Verification items for the finished model (mm, model axes). A direction names the side the tool comes from. Give positions to 0.01 mm unless a question says otherwise; leave off trailing zeros. Loops run counter-clockwise (first coordinate to the right, second up) from the corner with the lowest first, then second, coordinate; pieces in that order, holes last. Notation, with made-up numbers: (31, 12) - (51, 12) arc R22 cw to (51, 18) - close; hole circle Ø3 at (32, 88.5). An arc over 180 degrees is marked (long way). One line per question, with ' | ' between items. Start each with the question number.
1. Section check C-C, the plane y = 7. Enter the section's corners in (x, z).
2. Section check A-A, the plane y = 29. Enter the section's corners in (x, z).
3. Thickness scan on line 1 along Y through (x, z) = (38.5, 10.75); line 2 along Y through (x, z) = (47, 5.25); line 3 along X through (y, z) = (45.5, 11.25). Record the ranges inside material, lowest first. Write a range as from..to.
4. Tool access check on faces 4 (the face through (51, 18, 15)), 5 (the face through (39.8, 66, 11)), 6 (the face through (43, 10, 13)), 7 (the face through (-1, 31, 0)). Record the directions out of +Z, -Z, +X, -X, +Y, -Y that give a thin tool (end or side, any length) a straight path to the whole face; none if there is none.
5. Section check B-B, the plane x = 46.8. Enter the section's corners in (y, z), then the cut area to 3 significant figures.
6. Mould release check, pull along X, two halves, no side actions. Record for faces 1 (the face through (25, 67.23, 4.8)), 2 (the face through (55.8, 30.6, 4.8)), 3 (the face through (43, 25, 12)): +X half, -X half, draft (parallel to the pull), parting line (faces both ways), or undercut.
7. Depth check by flat-ended pin: pin 1 Ø5 at (x, y) = (2.5, 7.5) entering from +Z; pin 2 Ø15 at (x, y) = (33.5, 26) entering from +Z; pin 3 Ø5 at (x, y) = (45, 14) entering from +Z. Enter the tip coordinate at first touch or a pass-through.
8. Section check D-D, the plane x = 4. Enter the section's corners in (y, z).
from build123d import *

# Parameters (mm, degrees)
SKETCH_W        = 60.8
SKETCH_H        = 72.23
PAD_DEPTH       = 8
SKETCH001_R     = 3
PAD001_DEPTH    = 3
SKETCH002_W     = 50.8
SKETCH002_H     = 62.23
SKETCH002_R     = 3
POCKET_DEPTH    = 1
SKETCH003_W     = 60.8
SKETCH003_H     = 72.23
SKETCH003_W_2   = 54.8
SKETCH003_H_2   = 66.23
PAD002_DEPTH    = 18
SKETCH004_W     = 16
SKETCH004_H     = 13
POCKET001_DEPTH = 3.001
SKETCH005_W     = 8
SKETCH005_H     = 3
POCKET002_DEPTH = 3.001
SKETCH006_W     = 16
SKETCH006_H     = 5
POCKET003_DEPTH = 3
PAD003_DEPTH    = 32
SKETCH008_W     = 16
SKETCH008_H     = 3
POCKET004_DEPTH = 5
SKETCH009_W     = 2
SKETCH009_H     = 5
PAD004_DEPTH    = 20
SKETCH010_R     = 1
PAD005_DEPTH    = 2


with BuildPart() as part:
    # Sketch → Pad (new body)
    with BuildSketch(Plane.XY):
        with Locations((25.4, 31.115)):
            Rectangle(SKETCH_W, SKETCH_H)
    extrude(amount=-PAD_DEPTH)

    # Sketch001 (on Face5 of Pad) → Pad001 (join)
    with BuildSketch(Plane.XY):
        with Locations((46.8, 58.23)):
            Circle(SKETCH001_R)
        with Locations((4, 7)):
            Circle(SKETCH001_R)
    extrude(amount=PAD001_DEPTH)

    # Sketch002 (on Face4 of Pad001) → Pocket (cut)
    with BuildSketch(Plane.XY):
        with Locations((25.4, 31.115)):
            Rectangle(SKETCH002_W, SKETCH002_H)
        with Locations((46.8, 58.23)):
            Circle(SKETCH002_R, mode=Mode.SUBTRACT)
        with Locations((4, 7)):
            Circle(SKETCH002_R, mode=Mode.SUBTRACT)
    extrude(amount=-POCKET_DEPTH, mode=Mode.SUBTRACT)

    # Sketch003 (on Face4 of Pocket) → Pad002 (join)
    with BuildSketch(Plane.XY):
        with Locations((25.4, 31.115)):
            Rectangle(SKETCH003_W, SKETCH003_H)
        with Locations((25.4, 31.115)):
            Rectangle(SKETCH003_W_2, SKETCH003_H_2, mode=Mode.SUBTRACT)
    extrude(amount=PAD002_DEPTH)

    # Sketch004 (on Face11 of Pad002) → Pocket001 (cut, through all)
    with BuildSketch(Plane.XZ.offset(-64.23)):
        with Locations((31.8, 11.5)):
            Rectangle(SKETCH004_W, SKETCH004_H)
    extrude(amount=-POCKET001_DEPTH, mode=Mode.SUBTRACT)

    # Sketch005 (on Face17 of Pocket001) → Pocket002 (cut, through all)
    with BuildSketch(Plane(origin=(52.8, 0, 0), x_dir=(0, -1, 0), z_dir=(-1, 0, 0))):
        with Locations((-34.23, 6.5)):
            Rectangle(SKETCH005_W, SKETCH005_H)
    extrude(amount=-POCKET002_DEPTH, mode=Mode.SUBTRACT)

    # Sketch006 (on Face13 of Pocket002) → Pocket003 (cut)
    with BuildSketch(Plane.XZ.offset(5)):
        with Locations((42.8, 15.5)):
            Rectangle(SKETCH006_W, SKETCH006_H)
    extrude(amount=-POCKET003_DEPTH, mode=Mode.SUBTRACT)

    # Sketch007 (on Face21 of Pocket003) → Pad003 (join)
    with BuildSketch(Plane(origin=(0, -2, 0), x_dir=(-1, 0, 0), z_dir=(0, 1, 0))):
        Polygon((-50.8, 13), (-34.8, 13), (-34.8, 15), (-32.8, 15), (-32.8, 10), (-52.8, 10), (-52.8, 15), (-50.8, 15), align=None)
    extrude(amount=PAD003_DEPTH)

    # Sketch008 (on Face34 of Pad003) → Pocket004 (cut)
    with BuildSketch(Plane(origin=(0, 30, 0), x_dir=(-1, 0, 0), z_dir=(0, 1, 0))):
        with Locations((-42.8, 11.5)):
            Rectangle(SKETCH008_W, SKETCH008_H)
    extrude(amount=-POCKET004_DEPTH, mode=Mode.SUBTRACT)

    # Sketch009 (on Face25 of Pocket004) → Pad004 (join)
    with BuildSketch(Plane(origin=(52.8, 0, 0), x_dir=(0, -1, 0), z_dir=(-1, 0, 0))):
        with Locations((-31, 12.5)):
            Rectangle(SKETCH009_W, SKETCH009_H)
    extrude(amount=PAD004_DEPTH)

    # Sketch010 (on Face53 of Pad004) → Pad005 (join)
    with BuildSketch(Plane.XY.offset(3)):
        with Locations((46.8, 58.23)):
            Circle(SKETCH010_R)
        with Locations((4, 7)):
            Circle(SKETCH010_R)
    extrude(amount=PAD005_DEPTH)


solid = part.part
Results list:
1) outline: (-5, -8) - (55.8, -8) - (55.8, 18) - (52.8, 18) - (52.8, 15) - (50.8, 15) - (50.8, 13) - (34.8, 13) - (34.8, 15) - (32.8, 15) - (32.8, 10) - (52.8, 10) - (52.8, 0) - (50.8, 0) - (50.8, -1) - (7, -1) - (7, 3) - (5, 3) - (5, 5) - (3, 5) - (3, 3) - (1, 3) - (1, -1) - (0, -1) - (0, 0) - (-2, 0) - (-2, 18) - (-5, 18) - close
2) outline: (-5, -8) - (55.8, -8) - (55.8, 18) - (52.8, 18) - (52.8, 15) - (50.8, 15) - (50.8, 10) - (52.8, 10) - (52.8, 0) - (50.8, 0) - (50.8, -1) - (0, -1) - (0, 0) - (-2, 0) - (-2, 18) - (-5, 18) - close; (32.8, 10) - (34.8, 10) - (34.8, 15) - (32.8, 15) - close
3) line 1: -5..25, 30..32 | line 2: -5..-2, 64.23..67.23 | line 3: -5..-2, 52.8..55.8
4) face 4: +Z | face 5: +Z, +Y | face 6: +Z, -Y | face 7: none
5) outline: (-5, -8) - (67.23, -8) - (67.23, 18) - (64.23, 18) - (64.23, 0) - (62.23, 0) - (62.23, -1) - (61.23, -1) - (61.23, 3) - (59.23, 3) - (59.23, 5) - (57.23, 5) - (57.23, 3) - (55.23, 3) - (55.23, -1) - (0, -1) - (0, 0) - (-2, 0) - (-2, 10) - (25, 10) - (25, 13) - (-5, 13) - close; (30, 10) - (32, 10) - (32, 15) - (30, 15) - close | area: 728 mm²
6) face 1: draft | face 2: +X half | face 3: undercut
7) pin 1: z = 5 | pin 2: z = 15 | pin 3: z = 13
8) outline: (-5, -8) - (67.23, -8) - (67.23, 18) - (64.23, 18) - (64.23, 0) - (62.23, 0) - (62.23, -1) - (10, -1) - (10, 3) - (8, 3) - (8, 5) - (6, 5) - (6, 3) - (4, 3) - (4, -1) - (0, -1) - (0, 0) - (-2, 0) - (-2, 18) - (-5, 18) - close
